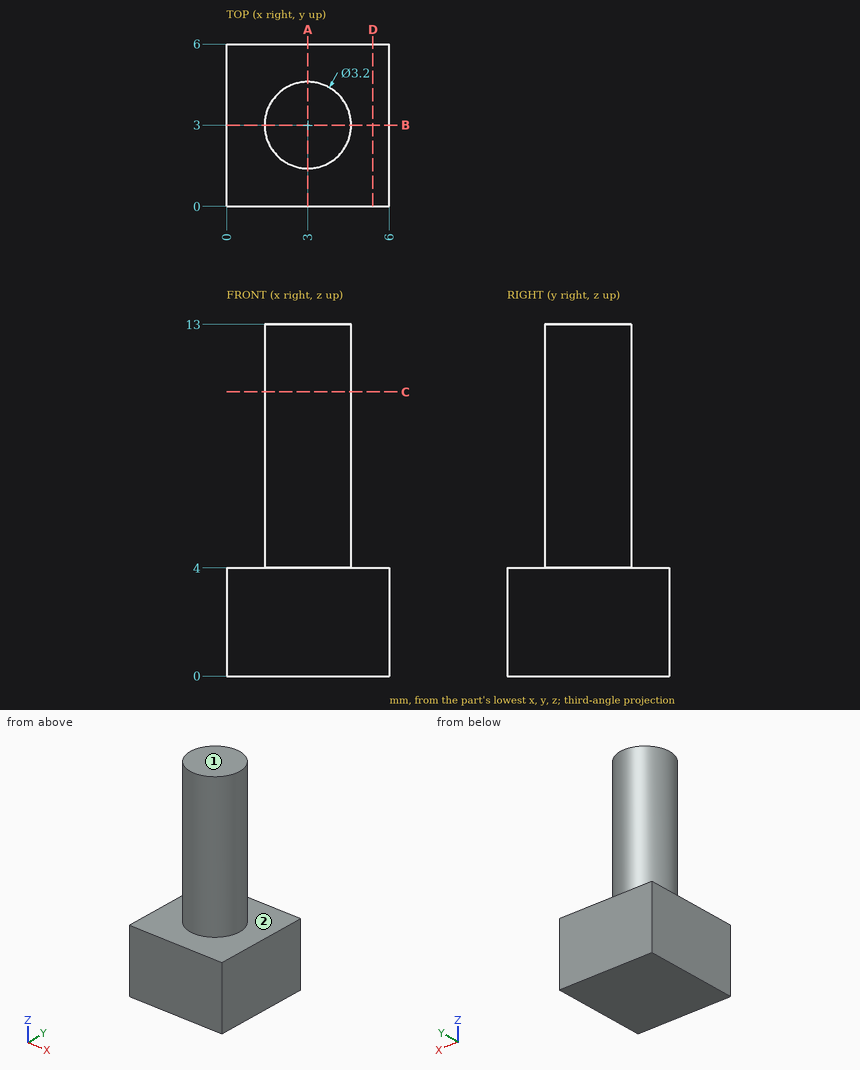
Verification items for this drawing (mm, ordinates from the low corner). A direction names the side the tool comes from. Coordinates: 2 decimals unless noted, no trailing zeros. Loops run counter-clockwise (first coordinate to the right, second up) from the corner with the lowest first, then second, coordinate; pieces in that order, holes last. Notation, with made-up numbers: (80.5, 18.5) -> (106.5, 18.5) arc R32 cw to (106.5, 44.5) -> close; hole circle Ø3 at (16.25, 40.5). An arc over 180 degrees is marked (long way). Answer in a Markdown table with one row per item. Add a question column.
1. Access from +Z, -Z, +X, -X, +Y, -Y to the whole of each face (thin tool, end or side, straight path). Record for the marked faces 1 and 2.
2. Section check C-C, the plane z = 10.5. Enter the section's corners in (x, y), then the cut area to 3 significant figures.
3. Section check A-A, the plane x = 3. Enter the section's corners in (y, z), then the cut area to 3 significant figures.
4. Material ranges on probe 1 along Z at (x, y) = (3.1, 0.9); probe 2 along Y at (x, z) = (2, 7); probe 3 along X at (y, z) = (3.55, 5), recorded low to high. Write a range as [from, to].
5. Section check D-D, the plane x = 5.4. Enter the section's corners in (y, z), then the cut area to 3 significant figures.
Derived:
| question | item | result |
|---|---|---|
| 1 | face 1 | +Z, +X, -X, +Y, -Y |
| 1 | face 2 | +Z |
| 2 | outline | circle Ø3.2 at (3, 3) |
| 2 | area | 8.04 mm² |
| 3 | outline | (0, 0) -> (6, 0) -> (6, 4) -> (4.6, 4) -> (4.6, 13) -> (1.4, 13) -> (1.4, 4) -> (0, 4) -> close |
| 3 | area | 52.8 mm² |
| 4 | probe 1 | z = [0, 4] |
| 4 | probe 2 | y = [1.75, 4.25] |
| 4 | probe 3 | x = [1.5, 4.5] |
| 5 | outline | (0, 0) -> (6, 0) -> (6, 4) -> (0, 4) -> close |
| 5 | area | 24.0 mm² |
